Study the drawing (mm; zero at the part's minimum x, y, z) and answer. A direction names the side the tool comes from. Round coordinates to 2 decimals unless told otherwise and drop trailing zeros. Loops run counter-clockwise (first coordinate to the right, second up) from the corner with the lowest first, then second, coordinate; pieces in that order, holes last. Notation, with made-up numbers: (17.5, -6) -> (33.5, -6) arc R31 ccw to (33.5, 20) -> close; hole circle Ø5 at (-30, 84). An arc over 180 degrees is marked (long way). Write each question's results on one line, items separated by ' | '. Start each with the question number.
(1) The part is cut by section A-A (z = 1.25). Determine the outline of the cut face in (x, y).
(2) Straight lines are drawn through the part: probe 1 along Z at (x, y) = (2.4, 3.8); probe 2 along Z at (x, y) = (4.3, 2.3); probe 3 along X at (y, z) = (0.8, 1) (1 decimal). For each, find the intervals that lie inside material, in ascending order.
(3) Determine the mould class of the marked faces 1, 2, 3 and 4 for opening direction Y: released by +Y, released by -Y, zero draft, split by the parting line, or undercut.
(4) For the marked faces 5, 6 and 7, determine the directions among +Z, -Z, +X, -X, +Y, -Y from which every point of the face is accessible in a straight line to the end or side of a thin tool.
(5) The part is cut by section B-B (y = 2.75). Determine the outline of the cut face in (x, z), plus the area to 3 significant figures.
(6) The part is cut by section C-C (z = 5). Determine the outline of the cut face in (x, y).
(7) Flat-ended cylindrical pins translate along their axes: pin 1 (2 mm diameter, centred on x = 0.5, z = 1, fed in from +Y); pin 2 (1 mm diameter, centred on x = 0.5, y = 4, fed in from +Z); pin 3 (1 mm diameter, centred on x = 1.5, z = 5, fed in from -Y). Find the tip coordinate at first contact, or state that the pin passes through.
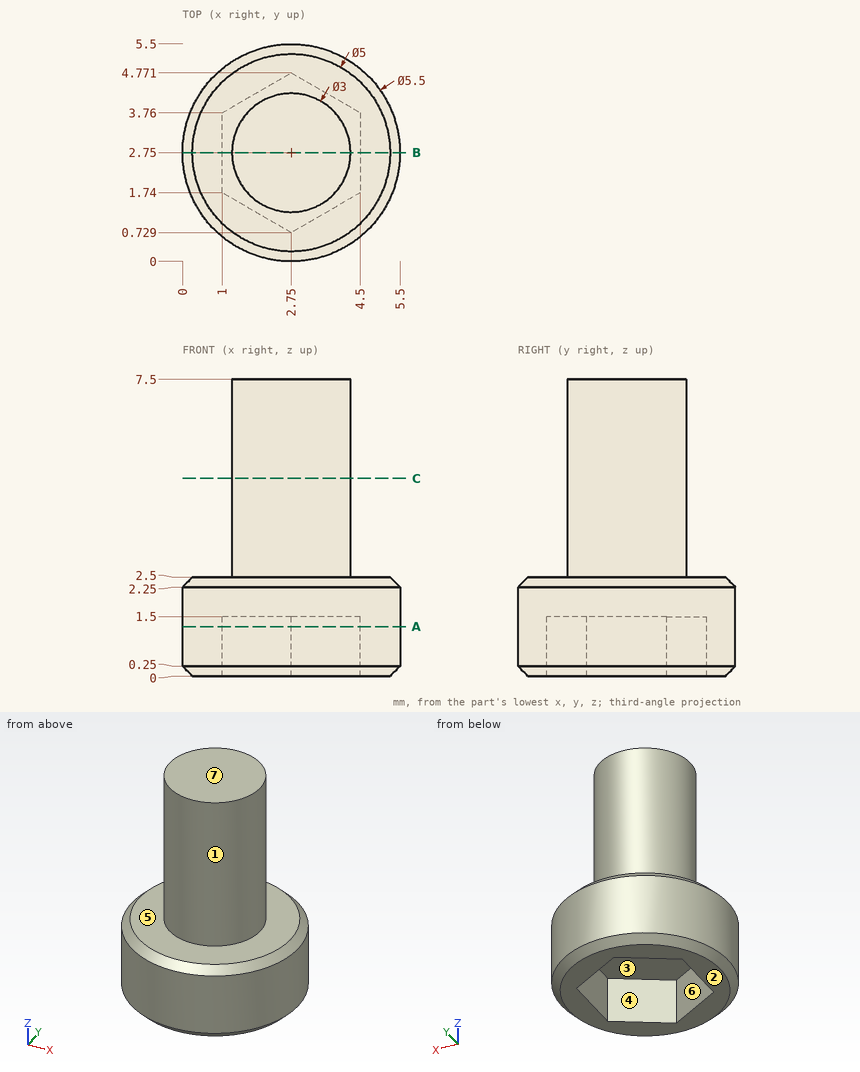
Checked values:
1) outline: circle Ø5.5 at (2.75, 2.75); hole (1, 1.74) -> (2.75, 0.73) -> (4.5, 1.74) -> (4.5, 3.76) -> (2.75, 4.77) -> (1, 3.76) -> close
2) probe 1: z = 1.5 to 7.5 | probe 2: z = 1.5 to 2.5 | probe 3: x = 0.8 to 2.6, 2.9 to 4.7
3) face 1: split by the parting line | face 2: zero draft | face 3: undercut | face 4: undercut
4) face 5: +Z | face 6: -Z | face 7: +Z, +X, -X, +Y, -Y
5) outline: (0, 0.25) -> (0.25, 0) -> (1, 0) -> (1, 1.5) -> (4.5, 1.5) -> (4.5, 0) -> (5.25, 0) -> (5.5, 0.25) -> (5.5, 2.25) -> (5.25, 2.5) -> (4.25, 2.5) -> (4.25, 7.5) -> (1.25, 7.5) -> (1.25, 2.5) -> (0.25, 2.5) -> (0, 2.25) -> close | area: 23.4 mm2
6) outline: circle Ø3 at (2.75, 2.75)
7) pin 1: stops at y = 5.2 | pin 2: stops at z = 2.5 | pin 3: stops at y = 1.45
